Autodesk Inventor part; units mm, degrees
ref_plane "Plano de trabalho1" through (20.3, 41, 0) normal (0, 0, -1) x (-1, 0, 0)
ref_plane "Plano de trabalho4" through (-89.9981, -8.0879, 0) normal (-1, 0, 0) x (0, 0, 1)
ref_plane "YZ Plane" through (0, 0, 0) normal (1, 0, 0) x (0, 1, 0)
ref_plane "Plano de trabalho1" through (20.3, 41, 0) normal (0, 0, -1) x (-1, 0, 0)
sketch "Esboço2" plane through (20.3, 41, 0) normal (0, 0, -1) x (-1, 0, 0)
  line L0 (-1, 1) -> (0, 0)
  line L1 (0, -40) -> (40.6, -40)
  line L2 (0, 0) -> (40.6, 0)
  line L3 (40.6, 0) -> (40.6, -40)
  line L4 (40.6, -40) -> (0, -40)
  line L5 (0, -40) -> (0, 0)
  circle A0 centre (20.3, -20) radius 4
  circle A1 centre (20.3, -20) radius 4
  circle A2 centre (20.3, -10.1005) radius 4
  circle A3 centre (20.3, -10.1005) radius 4
  circle A4 centre (20.3, -29.8995) radius 4
  circle A5 centre (20.3, -29.8995) radius 4
  circle A6 centre (25.2497, -5.1508) radius 1.1
  circle A7 centre (25.2497, -5.1508) radius 1.1
  circle A8 centre (25.2497, -15.0503) radius 1.1
  circle A9 centre (25.2497, -15.0503) radius 1.1
  circle A10 centre (25.2497, -24.9497) radius 1.1
  circle A11 centre (25.2497, -24.9497) radius 1.1
  circle A12 centre (25.2497, -34.8492) radius 1.1
  circle A13 centre (25.2497, -34.8492) radius 1.1
  circle A14 centre (33.8, -10) radius 1.1
  circle A15 centre (33.8, -10) radius 1.1
  circle A16 centre (33.8, -30) radius 1.1
  circle A17 centre (33.8, -30) radius 1.1
  circle A18 centre (33.8, -20) radius 1.1
  circle A19 centre (33.8, -20) radius 1.1
  circle A20 centre (15.3503, -5.1508) radius 1.1
  circle A21 centre (15.3503, -5.1508) radius 1.1
  circle A22 centre (15.3503, -15.0503) radius 1.1
  circle A23 centre (15.3503, -15.0503) radius 1.1
  circle A24 centre (15.3503, -24.9497) radius 1.1
  circle A25 centre (15.3503, -24.9497) radius 1.1
  circle A26 centre (15.3503, -34.8492) radius 1.1
  circle A27 centre (15.3503, -34.8492) radius 1.1
  circle A28 centre (6.8, -10) radius 1.1
  circle A29 centre (6.8, -10) radius 1.1
  circle A30 centre (6.8, -20) radius 1.1
  circle A31 centre (6.8, -20) radius 1.1
  circle A32 centre (6.8, -30) radius 1.1
  circle A33 centre (6.8, -30) radius 1.1
  line L6 (-1, 1) -> (41.6, 1)
  line L7 (41.6, 1) -> (41.6, -41)
  line L8 (41.6, -41) -> (-1, -41)
  line L9 (-1, -41) -> (-1, 1)
  line L10 (-1, 1) -> (41.6, -41) construction
  line L11 (41.6, 1) -> (-1, -41) construction
  line L12 (66.6981, -6.0879) -> (67.6981, -7.0879)
  line L13 (67.6981, -47.0879) -> (108.2981, -47.0879)
  line L14 (67.6981, -7.0879) -> (108.2981, -7.0879)
  line L15 (108.2981, -7.0879) -> (108.2981, -47.0879)
  line L16 (108.2981, -47.0879) -> (67.6981, -47.0879)
  line L17 (67.6981, -47.0879) -> (67.6981, -7.0879)
  circle A34 centre (87.9981, -27.0879) radius 4
  circle A35 centre (87.9981, -27.0879) radius 4
  circle A36 centre (87.9981, -17.1884) radius 4
  circle A37 centre (87.9981, -17.1884) radius 4
  circle A38 centre (87.9981, -36.9874) radius 4
  circle A39 centre (87.9981, -36.9874) radius 4
  circle A40 centre (92.9478, -12.2387) radius 1.1
  circle A41 centre (92.9478, -12.2387) radius 1.1
  circle A42 centre (92.9478, -22.1382) radius 1.1
  circle A43 centre (92.9478, -22.1382) radius 1.1
  circle A44 centre (92.9478, -32.0377) radius 1.1
  circle A45 centre (92.9478, -32.0377) radius 1.1
  circle A46 centre (92.9478, -41.9372) radius 1.1
  circle A47 centre (92.9478, -41.9372) radius 1.1
  circle A48 centre (101.4981, -17.0879) radius 1.1
  circle A49 centre (101.4981, -17.0879) radius 1.1
  circle A50 centre (101.4981, -37.0879) radius 1.1
  circle A51 centre (101.4981, -37.0879) radius 1.1
  circle A52 centre (101.4981, -27.0879) radius 1.1
  circle A53 centre (101.4981, -27.0879) radius 1.1
  circle A54 centre (83.0483, -12.2387) radius 1.1
  circle A55 centre (83.0483, -12.2387) radius 1.1
  circle A56 centre (83.0483, -22.1382) radius 1.1
  circle A57 centre (83.0483, -22.1382) radius 1.1
  circle A58 centre (83.0483, -32.0377) radius 1.1
  circle A59 centre (83.0483, -32.0377) radius 1.1
  circle A60 centre (83.0483, -41.9372) radius 1.1
  circle A61 centre (83.0483, -41.9372) radius 1.1
  circle A62 centre (74.4981, -17.0879) radius 1.1
  circle A63 centre (74.4981, -17.0879) radius 1.1
  circle A64 centre (74.4981, -27.0879) radius 1.1
  circle A65 centre (74.4981, -27.0879) radius 1.1
  circle A66 centre (74.4981, -37.0879) radius 1.1
  circle A67 centre (74.4981, -37.0879) radius 1.1
  line L18 (66.6981, -6.0879) -> (109.2981, -48.0879) construction
  line L19 (109.2981, -6.0879) -> (66.6981, -48.0879) construction
  line L20 (67.6981, -7.0879) -> (65.6981, -7.0879)
  line L21 (108.2981, -7.0879) -> (110.2981, -7.0879)
  line L22 (108.2981, -47.0879) -> (110.2981, -47.0879)
  line L23 (67.6981, -47.0879) -> (65.6981, -47.0879)
  line L24 (65.6981, -49.0879) -> (110.2981, -49.0879)
  line L25 (110.2981, -49.0879) -> (110.2981, -5.0879)
  line L26 (110.2981, -5.0879) -> (65.6981, -5.0879)
  line L27 (65.6981, -5.0879) -> (65.6981, -49.0879)
  line L28 (65.6981, -49.0879) -> (110.2981, -5.0879) construction
  line L29 (110.2981, -49.0879) -> (65.6981, -5.0879) construction
  point P0 (20.3, -41)
  point P1 (87.9981, -48.0879)
  dimension "d2" = 44.6
  dimension "d3" = 44
extrude "Extrusão1" add sketch "Esboço2" against normal blind 2 contours L17 L14 L15 L13
extrude "Extrusão2" add sketch "Esboço2" against normal blind 5 contours L13 L22 L25 L24 L27 L23 | L20 L27 L26 L25 L21 L14
extrude "Extrusão3" add sketch "Esboço2" against normal blind 14.04 contours L23 L27 L20 L17 | L15 L21 L25 L22
ref_plane "Plano de trabalho4" through (-89.9981, -8.0879, 0) normal (-1, 0, 0) x (0, 0, 1)
sketch "Esboço6" plane through (-89.9981, -8.0879, 0) normal (-1, 0, 0) x (0, 0, 1)
  circle A0 centre (9.54, 39.48) radius 1
  circle A1 centre (9.04, 25) radius 1
  circle A2 centre (9.54, 19.5) radius 1
  circle A3 centre (9, 4.5879) radius 1
  circle A4 centre (10.04, 12) radius 1
  line L0 (14.04, 35) -> (14.04, 42)
  line L1 (10.04, 35) -> (10.04, 27)
  line L2 (10.04, 35) -> (14.04, 39)
  line L3 (10.04, 27) -> (14.04, 23)
  line L4 (14.04, 39) -> (14.04, 23)
  line L5 (14.04, 42) -> (14.04, 2)
  point P0 (0, 8.0879)
  dimension "d12" = 2
  dimension "d14" = 2
  dimension "d17" = 2
  dimension "d19" = 2
  dimension "d21" = 2
  dimension "d24" = 4
  dimension "d26" = 8
extrude "Extrusão4" cut sketch "Esboço6" against normal blind 50 contours A0 | A1 | A2 | A3 | A4
extrude "Extrusão5" cut sketch "Esboço6" against normal blind 50 contours L4 L3 L1 L2 L0
properties part number "3 Cilindros"
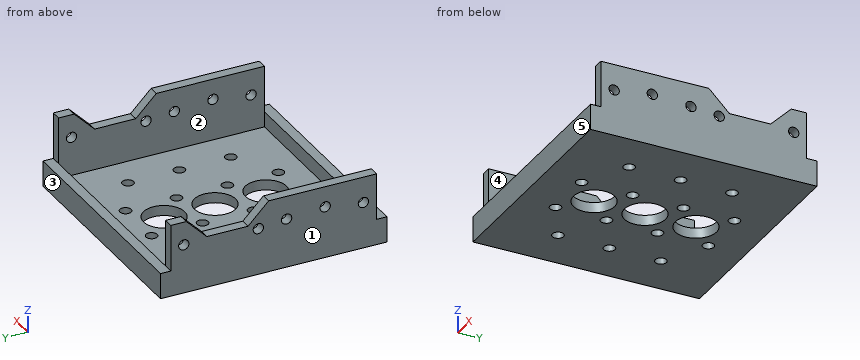
For this review, take the finished solid that the model builds, in its own axes (mm). Face numbers are marked on the shaded views. A direction names the side the tool comes from. Round coordinates to 2 decimals unless told otherwise and drop trailing zeros. Write each loop counter-clockwise with the first axis right and the second up, starting at its lowest first coordinate (ties: lowest second). Pieces come first, ordered by that corner, then holes. Notation, with made-up numbers: (48.5, -28.75) - (66.5, -28.75) arc R21 cw to (66.5, -14.75) - close; hole circle Ø11 at (54.25, 74). An arc over 180 degrees is marked (long way). Answer as CSV lines item,"result". Start each with the question number.
(1) Mouldability with a two-part tool opening along Y and no side actions: class the marked faces 3, 4 and 5 as +Y half, -Y half, draft (parallel to the pull), parting line (faces both ways), or undercut.
(2) Add section C-C, the plane z = 12.5. State the section outline as (x, y) points.
(3) Add section A-A, the plane z = 6. State the section outline as (x, y) points, plus the area to 3 significant figures.
(4) Add section D-D, the plane x = -77.5. State the section outline as (y, z) points, plus the area to 3 significant figures.
(5) Add section B-B, the plane y = -3.5. State the section outline as (x, z) points, plus the area to 3 significant figures.
(6) Machinability: for the marked faces 1 and 2, which of the approach directions +Z, -Z, +X, -X, +Y, -Y give a long, thin tool a straight path to every point of the face, cutting with its end or side? Answer none if there is none.
(7) For line 1 (X direction, y = 17, z = 5); line 2 (Y direction, x = -67, z = 3); line 3 (Y direction, x = -63.5, z = 1), list the stretches that pass through material, from the lowest coordinate up.
(8) For pin 1 (20 mm diameter, centred on x = -69, y = 10.5, fed in from +Z); pin 2 (2 mm diameter, centred on x = -79, y = -7.5, fed in from +Z); pin 3 (2 mm diameter, centred on x = -47, z = 11, fed in from +Y), all flat-tipped, find the tip position at first contact; note any pin that passes through.
From the geometry:
1,face 3,"+Y half"
1,face 4,"undercut"
1,face 5,"-Y half"
2,outline,"(-90, -6.09) - (-88, -6.09) - (-88, 16.45) - (-90, 16.45) - close; (-90, 29.37) - (-88, 29.37) - (-88, 33.91) - (-90, 33.91) - close; (-47.4, -6.09) - (-45.4, -6.09) - (-45.4, 16.45) - (-47.4, 16.45) - close; (-47.4, 29.37) - (-45.4, 29.37) - (-45.4, 33.91) - (-47.4, 33.91) - close"
3,outline,"(-90, -6.09) - (-88, -6.09) - (-88, 33.91) - (-90, 33.91) - close; (-47.4, -6.09) - (-45.4, -6.09) - (-45.4, 33.91) - (-47.4, 33.91) - close"
3,area,"160 mm²"
4,outline,"(-8.09, 0) - (35.91, 0) - (35.91, 5) - (33.91, 5) - (33.91, 2) - (-6.09, 2) - (-6.09, 5) - (-8.09, 5) - close"
4,area,"100 mm²"
5,outline,"(-90, 0) - (-45.4, 0) - (-45.4, 8) - (-47.4, 8) - (-47.4, 2) - (-88, 2) - (-88, 8) - (-90, 8) - close; (-90, 10) - (-88, 10) - (-88, 14.04) - (-90, 14.04) - close; (-47.4, 10) - (-45.4, 10) - (-45.4, 14.04) - (-47.4, 14.04) - close"
5,area,"129 mm²"
6,face 1,"+Z, -Z, -X, +Y, -Y"
6,face 2,"+Z"
7,line 1,"x = -90 to -88, -47.4 to -45.4"
7,line 2,"y = -8.09 to -6.09, 33.91 to 35.91"
7,line 3,"y = -8.09 to -1.74, -0.13 to 8.16, 9.77 to 18.06, 19.66 to 27.96, 29.56 to 35.91"
8,pin 1,"stops at z = 2"
8,pin 2,"stops at z = 5"
8,pin 3,"stops at y = 33.91"
